The listing builds one solid part. Answer for the finished solid, in the listing's coordinates (mm). A direction names the side the tool comes from. Give positions to 0.01 mm unless a question says otherwise; leave off trailing zeros. Write each loop counter-clockwise with the first axis right and the second up, starting at its lowest first coordinate (ties: lowest second). Pieces come first, ordered by that corner, then holes. Notation, with made-up numbers: M -2.75,57.5 L 24.25,57.5 A33 cw 24.25,88.5 Z; hole C 77,-36.5 d1. An arc over 180 degrees is marked long. Return JSON: item names as keys, results as strings.
from build123d import *

# Parameters (mm, degrees)
F1_DEPTH = 3
F2_W     = 1.4
F2_H     = 1.4
F3_DEPTH = 1.2
F4_R     = 0.5
F5_R     = 0.2
F6_W     = 0.8
F6_H     = 1
F7_DEPTH = 8


with BuildPart() as f1:
    # F0 (on Top) → F1 (new body)
    with BuildSketch(Plane.XY):
        Polygon((0, 0.8), (0, 0), (8, 0), (8, 0.8), (5.5, 0.8), (5.5, 3.3), (2.5, 3.3), (2.5, 0.8), align=None)
    extrude(amount=F1_DEPTH)

    # F2 (on face) → F3 (cut)
    with BuildSketch(Plane.XZ):
        with Locations((4, 1.5)):
            Rectangle(F2_W, F2_H)
    extrude(amount=-F3_DEPTH, mode=Mode.SUBTRACT)

    # F4
    f4_edges = [f1.edges().sort_by_distance(p)[0] for p in [
        (5.5, 2.05, 3),
        (2.5, 2.05, 3),
        (2.5, 2.05, 0),
        (5.5, 2.05, 0),
    ]]
    fillet(f4_edges, radius=F4_R)

    # F5
    f5_edges = [f1.edges().sort_by_distance(p)[0] for p in [
        (4, 3.3, 3),
        (5.353553, 3.3, 2.853553),
        (5.5, 3.3, 1.5),
        (5.353553, 3.3, 0.146447),
        (4, 3.3, 0),
        (2.646447, 3.3, 0.146447),
        (2.5, 3.3, 1.5),
        (2.646447, 3.3, 2.853553),
    ]]
    fillet(f5_edges, radius=F5_R)

    # F6 (on face) → F7 (join, through all)
    with BuildSketch(Plane.YZ.offset(8)):
        with Locations((0.4, 3.5)):
            Rectangle(F6_W, F6_H)
    extrude(amount=-F7_DEPTH)


solid = f1.part
Item 1: A cutting plane is placed at B-B, the plane z = 1.05. Write down the section's boundary in (x, y).
Geometry results:
{"outline": "M 0,0 L 3.3,0 L 3.3,1.2 L 4.7,1.2 L 4.7,0 L 8,0 L 8,0.8 L 5.5,0.8 L 5.5,3.1 A0.2 ccw 5.3,3.3 L 2.7,3.3 A0.2 ccw 2.5,3.1 L 2.5,0.8 L 0,0.8 Z"}
Item 2: Which of the six approach directions +Z, -Z, +X, -X, +Y, -Y give full straight-line access (tool end or side, diameter ignored) to faces 1 (the flat face through (4, 2, 3)), 2 (the flat face through (2.5, 2, 1)), 3 (the flat face through (4, 3.3, 1)), 4 (the flat face through (3.3, 1, 1)), 5 (the flat face through (4.1, 0, 2.4))?
Geometry results:
{"face 1": "+Z, +X, -X, +Y", "face 2": "+Z, -Z, -X, +Y", "face 3": "+Z, -Z, +X, -X, +Y", "face 4": "-Y", "face 5": "+Z, -Z, +X, -X, -Y"}
Item 3: Find the intervals of material crossed by line 1 (X direction, y = 0.55, z = 0.95); line 2 (Y direction, x = 0.75, z = 3.3); line 3 (Z direction, x = 5, y = 1.05), in increasing order.
Geometry results:
{"line 1": "x = 0 to 3.3, 4.7 to 8", "line 2": "y = 0 to 0.8", "line 3": "z = 0 to 3"}
Item 4: A cutting plane is placed at A-A, the plane y = 0.55. Write down the section's boundary in (x, z).
Geometry results:
{"outline": "M 0,0 L 8,0 L 8,4 L 0,4 Z; hole M 3.3,0.8 L 4.7,0.8 L 4.7,2.2 L 3.3,2.2 Z"}
Item 5: A cutting plane is placed at D-D, the plane x = 4. Write down the section's boundary in (y, z).
Geometry results:
{"outline": "M 0,0 L 3.1,0 A0.2 ccw 3.3,0.2 L 3.3,2.8 A0.2 ccw 3.1,3 L 0.8,3 L 0.8,4 L 0,4 L 0,2.2 L 1.2,2.2 L 1.2,0.8 L 0,0.8 Z"}
Item 6: Determine the mould class of faces 6 (the flat face through (4, 1, 0.8)), 7 (the flat face through (5.5, 2, 1)), 8 (the flat face through (4.1, 0.8, 3.3)) for opening direction X: +X half, -X half, draft (parallel to the pull), parting line (faces both ways), or undercut.
Geometry results:
{"face 6": "undercut", "face 7": "+X half", "face 8": "draft"}
Item 7: Given pin 1 Ø1.5 at (x, y) = (5.5, 2) entering from -Z; pin 2 Ø1 at (y, z) = (1.5, 1.5) entering from +X; pin 3 Ø0.7 at (x, z) = (4, 1.5) entering from -Y, each flat-ended and moving along its own axis, determine where each tip first touches the part or whether it passes through.
Geometry results:
{"pin 1": "stops at z = 0", "pin 2": "stops at x = 5.5", "pin 3": "stops at y = 1.2"}
Item 8: A cutting plane is placed at C-C, the plane y = 1.9. Write down the section's boundary in (x, z).
Geometry results:
{"outline": "M 2.5,0.5 A0.5 ccw 3,0 L 5,0 A0.5 ccw 5.5,0.5 L 5.5,2.5 A0.5 ccw 5,3 L 3,3 A0.5 ccw 2.5,2.5 Z"}
